Geometry: final body of the model. Coordinates: model frame, mm. A direction names the side the tool comes from. Give positions to 0.01 mm unless a question says otherwise; leave off trailing zeros. Order: outer loops, then holes, each group sorted by start corner. A loop starts at its lowest first (then second) coordinate and runs counter-clockwise, first axis right, second up. Notation, with made-up numbers: (79.25, -13.75) - (97.25, -13.75) arc R9 ccw to (97.25, 1.25) - close; hole circle Ø4 at (-4, -10.5). An arc over 180 degrees is marked (long way). Use one line per item in the form item = value.
from build123d import *
from build123d.topology import SkipClean

# Parameters (mm, degrees)
SKETCH1_R           = 4
BOSS_EXTRUDE1_DEPTH = 6
SKETCH2_R           = 12
BOSS_EXTRUDE2_DEPTH = 6
SKETCH3_R           = 18
SKETCH3_R_2         = 12
BOSS_EXTRUDE3_DEPTH = 14
FILLET1_R           = 4
BOSS_EXTRUDE4_START = -4
BOSS_EXTRUDE4_DEPTH = 4


with BuildPart() as part:
    # Sketch1 → Boss-Extrude1 (new body)
    with BuildSketch(Plane(origin=(0, 0, 0), x_dir=(1, 0, 0), z_dir=(0, 1, 0))):
        with BuildLine():
            Line((-30, 18), (22, 18))
            ThreePointArc((22, 18), (27.656854249, 15.656854249), (30, 10))
            Line((30, 10), (30, -10))
            ThreePointArc((30, -10), (27.656854249, -15.656854249), (22, -18))
            Line((22, -18), (-30, -18))
            Line((-30, -18), (-30, 18))
        make_face()
        with Locations(Location((22, -10, 0), (0, 0, 270))):
            Circle(SKETCH1_R, mode=Mode.SUBTRACT)
        with Locations(Location((22, 10, 0), (0, 0, 90))):
            Circle(SKETCH1_R, mode=Mode.SUBTRACT)
        with BuildLine():
            Line((-1, 4), (7, 4))
            ThreePointArc((7, 4), (11, 0), (7, -4))
            Line((7, -4), (-1, -4))
            ThreePointArc((-1, -4), (-5, 0), (-1, 4))
        make_face(mode=Mode.SUBTRACT)
    extrude(amount=BOSS_EXTRUDE1_DEPTH)

    # Sketch2 → Boss-Extrude2 (add)
    with BuildSketch(Plane.ZY.offset(30)):
        with BuildLine():
            Line((-18, 0), (-18, 30))
            ThreePointArc((-18, 30), (0, 48), (18, 30))
            Line((18, 30), (18, 0))
            Line((18, 0), (-18, 0))
        make_face()
        with Locations((0, 30)):
            Circle(SKETCH2_R, mode=Mode.SUBTRACT)
    extrude(amount=BOSS_EXTRUDE2_DEPTH)

    # Sketch3 → Boss-Extrude3 (add)
    with SkipClean():  # the faces are left unmerged after this step: merging them gives an invalid solid
        with BuildSketch(Plane.ZY.offset(36)):
            with Locations((0, 30)):
                Circle(SKETCH3_R)
            with Locations((0, 30)):
                Circle(SKETCH3_R_2, mode=Mode.SUBTRACT)
        extrude(amount=BOSS_EXTRUDE3_DEPTH)
    add(part.part.scale(1), mode=Mode.REPLACE)  # the faces are merged on a copy

    # Fillet1
    fillet1_edges = [part.edges().sort_by_distance(p)[0] for p in [
        (-30, 6, 0),
    ]]
    fillet(fillet1_edges, radius=FILLET1_R)

    # Sketch4 → Boss-Extrude4 (add)
    with BuildSketch(Plane.XY.offset(15).offset(BOSS_EXTRUDE4_START)):
        with BuildLine():
            Line((-26, 6), (-12, 6))
            Line((-12, 6), (-30, 24))
            Line((-30, 24), (-30, 10))
            ThreePointArc((-30, 10), (-28.828427125, 7.171572875), (-26, 6))
        make_face()
    boss_extrude4 = extrude(amount=BOSS_EXTRUDE4_DEPTH)

    # Mirror1: Boss-Extrude4 across plane
    add(boss_extrude4.mirror(Plane(origin=(0, 0, 0), x_dir=(1, 0, 0), z_dir=(0, 0, -1))))


solid = part.part
(1) Ray query, line 1 along Y through (x, z) = (-39.5, 0); line 2 along X through (y, z) = (3, -10); line 3 along Y through (x, z) = (12.5, -1). Return the intervals inside material, ascending.
Computed values:
line_1 = 12 to 18, 42 to 48
line_2 = -36 to 18, 26 to 30
line_3 = 0 to 6
(2) Cut plane D-D on x = 8. Output: boundary loops of the cut face in (y, z).
Computed values:
outline = (0, -18) - (6, -18) - (6, -3.87) - (0, -3.87) - close; (0, 3.87) - (6, 3.87) - (6, 18) - (0, 18) - close
(3) Contact query for flat-ended pins moving along their axis: pin 1 Ø6.5 at (x, z) = (22, -10) entering from +Y; pin 2 Ø5 at (x, y) = (-17, 7.5) entering from -Z; pin 3 Ø9 at (x, z) = (22, 10) entering from +Y; pin 4 Ø14.5 at (x, y) = (-21, 17) entering from -Z. Output: stop coordinate, or through.
Computed values:
pin_1 = through
pin_2 = -18
pin_3 = 6
pin_4 = -15
(4) Cut plane A-A on y = 40.5. Output: boundary loops of the cut face in (x, z).
Computed values:
outline = (-50, -14.62) - (-30, -14.62) - (-30, -5.81) - (-50, -5.81) - close; (-50, 5.81) - (-30, 5.81) - (-30, 14.62) - (-50, 14.62) - close
(5) Cut plane B-B on x = -22. Output: boundary loops of the cut face in (y, z).
Computed values:
outline = (0, -18) - (6, -18) - (6, -15) - (16, -15) - (16, -11) - (6, -11) - (6, 11) - (16, 11) - (16, 15) - (6, 15) - (6, 18) - (0, 18) - close
(6) Pull-direction query (Y, two-part tool) for faces 1 (the face through (-39.86, 30.53, -11.99)), 2 (the face through (-28.859, 7.203, -0.154)), 3 (the face through (-36, 9, 0)); classes: released by +Y, released by -Y, zero draft, split by the parting line, or undercut.
Computed values:
face_1 = undercut
face_2 = released by +Y
face_3 = zero draft
(7) Reachability of faces 4 (the face through (-25, 11, 15)), 5 (the face through (-25, 11, -15)), 6 (the face through (-30, 20.8, 8.3)) from +Z, -Z, +X, -X, +Y, -Y: full face, straight path, thin tool, end or side. Return the list, or none.
Computed values:
face_4 = +Z, +X, +Y
face_5 = -Z, +X, +Y
face_6 = +X, +Y
(8) Cut plane C-C on z = 2. Output: boundary loops of the cut face in (x, y).
Computed values:
outline = (-50, 12.11) - (-36, 12.11) - (-36, 0) - (-4.46, 0) - (-4.46, 6) - (-26, 6) arc R4 cw to (-30, 10) - (-30, 18.17) - (-50, 18.17) - close; (-50, 41.83) - (-30, 41.83) - (-30, 47.89) - (-50, 47.89) - close; (10.46, 0) - (30, 0) - (30, 6) - (10.46, 6) - close
